Source: CAD feature listing. Evaluate the final solid. Frame: model axes, mm. A direction names the side the tool comes from. Round coordinates to 2 decimals unless told otherwise and drop trailing zeros. Order: outer loops, then holes, each group sorted by start corner. A loop starts at its lowest first (then second) coordinate and runs counter-clockwise, first axis right, second up. Notation, with made-up numbers: (4.5, -15.75) -> (27.5, -15.75) arc R11 cw to (27.5, -11.75) -> close; hole circle Ø11 at (43, 6.5). An arc over 180 degrees is marked (long way). Write item = value, one per line. Start each with the question number.
(1) Cut plane A-A on y = -12.5. Return the cut outline in (x, z), then the cut area to 3 significant figures.
(2) Reachability of faces 1 (the face through (-4.386, -12, 19)), 2 (the face through (4.386, -12, 19)), 3 (the face through (0, -17.545, 19)), 4 (the face through (0, 17.545, 19)), 5 (the face through (-8.4, 0.1, 19)) from +Z, -Z, +X, -X, +Y, -Y: full face, straight path, thin tool, end or side. Return the list, or none.
(3) Contact query for flat-ended pins moving along their axis: pin 1 Ø1.5 at (x, y) = (-9, -7.5) entering from -Z; pin 2 Ø3 at (y, z) = (-11.5, 19) entering from -X; pin 3 Ø2 at (x, y) = (-11, 9) entering from +Z; pin 4 Ø5 at (y, z) = (-13, 18) entering from +X. Output: stop coordinate, or through.
(4) Cut plane D-D on y = 19. Return the cut outline in (x, z), then the cut area to 3 significant figures.
(5) Ray query, line 1 (Z direction, x = 16, y = 33); line 2 (Y direction, x = -2, z = 15.25); line 3 (X direction, y = 11.5, z = 19.25). Return the intervals inside material, ascending.
(6) Cut plane C-C on x = -14. Return the cut outline in (y, z).
(7) Cut plane B-B on z = 13.5. Return the cut outline in (x, y), then the cut area to 3 significant figures.
from build123d import *

# Parameters (mm, degrees)
F1_DEPTH = 25.4
F0_W     = 51.7266914248
F0_H     = 71.9938799739
F2_DEPTH = 12.7


with BuildPart() as f1:
    # F0 (on Top) → F1 (new body)
    with BuildSketch(Plane.XY):
        with BuildLine():
            ThreePointArc((4.3861824088, -7.1647320158), (7.3286779539, -4.1063926297), (8.4007131233, 0))
            ThreePointArc((8.4007131233, 0), (7.3286779539, 4.1063926297), (4.3861824088, 7.1647320158))
            Line((4.3861824088, 7.1647320158), (4.3861824088, -7.1647320158))
        make_face()
        with BuildLine():
            Line((4.3861824088, -7.1647320158), (4.3861824088, 7.1647320158))
            ThreePointArc((4.3861824088, 7.1647320158), (0, 8.4007131233), (-4.3861824088, 7.1647320158))
            Line((-4.3861824088, 7.1647320158), (-4.3861824088, -7.1647320158))
            ThreePointArc((-4.3861824088, -7.1647320158), (0, -8.4007131233), (4.3861824088, -7.1647320158))
        make_face()
        with BuildLine():
            Line((-4.3861824088, -7.1647320158), (-4.3861824088, 7.1647320158))
            ThreePointArc((-4.3861824088, 7.1647320158), (-8.4007131233, 0), (-4.3861824088, -7.1647320158))
        make_face()
        with BuildLine():
            Line((4.3861824088, -17.5447259098), (4.3861824088, -7.1647320158))
            ThreePointArc((4.3861824088, -7.1647320158), (0, -8.4007131233), (-4.3861824088, -7.1647320158))
            Line((-4.3861824088, -7.1647320158), (-4.3861824088, -17.5447259098))
            Line((-4.3861824088, -17.5447259098), (4.3861824088, -17.5447259098))
        make_face()
        with BuildLine():
            ThreePointArc((-4.3861824088, 7.1647320158), (0, 8.4007131233), (4.3861824088, 7.1647320158))
            Line((4.3861824088, 7.1647320158), (4.3861824088, 17.5447259098))
            Line((4.3861824088, 17.5447259098), (-4.3861824088, 17.5447259098))
            Line((-4.3861824088, 17.5447259098), (-4.3861824088, 7.1647320158))
        make_face()
    extrude(amount=F1_DEPTH)

    # F0 (on Top) → F2 (join)
    with BuildSketch(Plane.XY):
        Rectangle(F0_W, F0_H)
        with BuildLine():
            ThreePointArc((4.3861824088, 7.1647320158), (7.3286779539, 4.1063926297), (8.4007131233, 0))
            ThreePointArc((8.4007131233, 0), (7.3286779539, -4.1063926297), (4.3861824088, -7.1647320158))
            Line((4.3861824088, -7.1647320158), (4.3861824088, -17.5447259098))
            Line((4.3861824088, -17.5447259098), (-4.3861824088, -17.5447259098))
            Line((-4.3861824088, -17.5447259098), (-4.3861824088, -7.1647320158))
            ThreePointArc((-4.3861824088, -7.1647320158), (-8.4007131233, 0), (-4.3861824088, 7.1647320158))
            Line((-4.3861824088, 7.1647320158), (-4.3861824088, 17.5447259098))
            Line((-4.3861824088, 17.5447259098), (4.3861824088, 17.5447259098))
            Line((4.3861824088, 17.5447259098), (4.3861824088, 7.1647320158))
        make_face(mode=Mode.SUBTRACT)
    extrude(amount=F2_DEPTH)


solid = f1.part
Evaluation:
q1.outline = (-25.86, 0) -> (25.86, 0) -> (25.86, 12.7) -> (4.39, 12.7) -> (4.39, 25.4) -> (-4.39, 25.4) -> (-4.39, 12.7) -> (-25.86, 12.7) -> close
q1.area = 768 mm^2
q2.face_1 = +Z, -X, -Y
q2.face_2 = +Z, +X, -Y
q2.face_3 = +Z, +X, -X, -Y
q2.face_4 = +Z, +X, -X, +Y
q2.face_5 = +Z, -X
q3.pin_1 = 0
q3.pin_2 = -4.39
q3.pin_3 = 12.7
q3.pin_4 = 4.39
q4.outline = (-25.86, 0) -> (25.86, 0) -> (25.86, 12.7) -> (-25.86, 12.7) -> close
q4.area = 657 mm^2
q5.line_1 = 0 to 12.7
q5.line_2 = -17.54 to 17.54
q5.line_3 = -4.39 to 4.39
q6.outline = (-36, 0) -> (36, 0) -> (36, 12.7) -> (-36, 12.7) -> close
q7.outline = (-4.39, -17.54) -> (4.39, -17.54) -> (4.39, -7.16) arc R8.4 ccw to (4.39, 7.16) -> (4.39, 17.54) -> (-4.39, 17.54) -> (-4.39, 7.16) arc R8.4 ccw to (-4.39, -7.16) -> close
q7.area = 389 mm^2
